Autodesk Inventor part; units mm, degrees
ref_plane "YZ Plane" through (0, 0, 0) normal (1, 0, 0) x (0, 1, 0)
ref_plane "XZ Plane" through (0, 0, 0) normal (0, 1, 0) x (-1, 0, 0)
ref_plane "XY Plane" through (0, 0, 0) normal (0, 0, 1) x (1, 0, 0)
sketch "Sketch2" plane through (0, 0, 0) normal (0, 0, 1) x (1, 0, 0)
  arc A0 (0, -52) -> (0, 52) centre (0, 0) ccw
  arc A1 (0, -50) -> (0, 50) centre (0, 0) ccw
  line L0 (0, 52) -> (0, 50)
  line L1 (0, -50) -> (0, -52)
  line L2 (2, 49.96) -> (4, 49.96)
  line L3 (4, 49.96) -> (4, 65.96)
  line L4 (4, 65.96) -> (2, 65.96)
  line L5 (2, 65.96) -> (2, 49.96)
  line L6 (2, -49.96) -> (4, -49.96)
  line L7 (4, -49.96) -> (4, -65.96)
  line L8 (4, -65.96) -> (2, -65.96)
  line L9 (2, -65.96) -> (2, -49.96)
  line L10 (0, 92.344) -> (0, -92.344) construction
  point P0 (4, -51.8459)
  point P1 (4, 51.8459)
  dimension "d0" = 104
  dimension "d1" = 100
  dimension "d2" = 2
  dimension "d40" = 2
  dimension "d41" = 2
  dimension "d42" = 16
  dimension "d43" = 16
  dimension "d44" = 2
  dimension "d45" = 2
extrude "Extrusion1" add sketch "Sketch2" along normal blind 80 contours L9 L6 L7 A0 | A0 L7 L8 L9 | L7 L6 A1 L2 L3 A0 | L3 L2 L5 A0 | A0 L5 L4 L3
fillet "Fillet4" radius 2 2 edges at (4, 51.8459, 40) (4, -51.8459, 40)
sketch "Sketch6" plane through (4, -65.96, 80) normal (1, 0, 0) x (0, 0, -1)
  line L0 (80, 16) -> (80, 0) construction
  line L1 (80, 0) -> (0, 0) construction
  line L2 (0, 16) -> (0, 0) construction
  line L3 (80, 16) -> (0, 16) construction
  line L4 (80, 131.92) -> (80, 115.92) construction
  line L5 (80, 115.92) -> (0, 115.92) construction
  line L6 (0, 131.92) -> (0, 115.92) construction
  line L7 (80, 131.92) -> (0, 131.92) construction
  point P0 (80, 65.96)
  point P1 (15, 6)
  point P2 (65, 6)
  point P3 (65, 125.92)
  point P4 (15, 125.92)
  dimension "d47" = 15
  dimension "d48" = 15
  dimension "d49" = 15
  dimension "d50" = 15
  dimension "d51" = 6
  dimension "d52" = 6
  dimension "d53" = 6
  dimension "d54" = 6
hole "Hole3" at (4, -59.96, 65) at (4, -59.96, 15) at (4, 59.96, 15) at (4, 59.96, 65) direction (-1, 0, 0) diameter 6.5 depth 2
properties part number "P050_SupportTube2"
For this review, take the finished solid that the model builds, in its own axes (mm). A direction names the side the tool comes from. Round coordinates to 2 decimals unless told otherwise and drop trailing zeros. Write each loop counter-clockwise with the first axis right and the second up, starting at its lowest first coordinate (ties: lowest second). Pieces come first, ordered by that corner, then holes. Notation, with made-up numbers: M 83,76 L 96,76 A24 cw 96,86 Z; hole C 54,70.5 d5. An arc over 180 degrees is marked long. One line per item, written item: value. Start each with the question number.
(1) We need section B-B (y = 59.96). Give the boundary of the cut face in (x, z), and give its area (3 significant figures).
(2) Insertion check: pin 1 (4 mm diameter, centred on x = 45.5, z = 17.5, fed in from +Y); pin 2 (1 mm diameter, centred on x = 46.5, z = 18.5, fed in from -Y); pin 3 (1 mm diameter, centred on y = 35.5, z = 45, fed in from +X). Each pin has a flat end and moves straight along its axis. Give the tip position at first contact, or say it passes through.
(3) We need section D-D (z = 24.5). Give the boundary of the cut face in (x, y).
(4) Wall thickness on line 1 (Z direction, x = 3.55, y = -59.96); line 2 (Y direction, x = 3.4, z = 15); line 3 (X direction, y = 53.5, z = 22.5): over which ranges is each line inside the solid? List them lowest first.
(5) Machinability: for faces 5 (the flat face through (4, -60, 39)), 6 (the cylindrical face through (2.986, -60.103, 68.247)), 7 (the flat face through (4, 60, 39)), which of the approach directions +Z, -Z, +X, -X, +Y, -Y give a long, thin tool a straight path to every point of the face, cutting with its end or side? Answer none if there is none.
(6) We need section C-C (z = 65). Give the boundary of the cut face in (x, y).
(7) We need section A-A (x = 48). Give the boundary of the cut face in (y, z), and give its area (3 significant figures).
(8) The part is to be moulded in two halves that separate along Y. For faces 1 (the cylindrical face through (49.99, 1.07, 39.44)), 2 (the flat face through (51, 0, 80)), 3 (the cylindrical face through (2.986, -62.157, 17.395)), 4 (the cylindrical face through (51.99, 1.06, 39.44)), say which applies: released by +Y, released by -Y, zero draft, split by the parting line, or undercut.
Result:
1. outline: M 2,0 L 4,0 L 4,11.75 L 2,11.75 Z; M 2,18.25 L 4,18.25 L 4,61.75 L 2,61.75 Z; M 2,68.25 L 4,68.25 L 4,80 L 2,80 Z
1. area: 134 mm²
2. pin 1: y = 28.49
2. pin 2: y = -24.25
2. pin 3: x = 38.46
3. outline: M 2,-65.96 L 4,-65.96 L 4,-53.67 A2 cw 5.78,-51.68 A52 ccw 5.78,51.68 A2 cw 4,53.67 L 4,65.96 L 2,65.96 L 2,49.96 A50 cw 2,-49.96 Z
4. line 1: 0 to 11.75, 18.25 to 61.75, 68.25 to 80
4. line 2: -65.96 to -63.21, -56.71 to -49.88, 49.88 to 56.71, 63.21 to 65.96
4. line 3: 2 to 4.01
5. face 5: +Z, -Z, +X, -Y
5. face 6: +X, -X
5. face 7: +Z, -Z, +X, +Y
6. outline: M 2,-65.96 L 4,-65.96 L 4,-63.21 L 2,-63.21 Z; M 2,-56.71 L 4,-56.71 L 4,-53.67 A2 cw 5.78,-51.68 A52 ccw 5.78,51.68 A2 cw 4,53.67 L 4,56.71 L 2,56.71 L 2,49.96 A50 cw 2,-49.96 Z; M 2,63.21 L 4,63.21 L 4,65.96 L 2,65.96 Z
7. outline: M -20,0 L -14,0 L -14,80 L -20,80 Z; M 14,0 L 20,0 L 20,80 L 14,80 Z
7. area: 960 mm²
8. face 1: undercut
8. face 2: zero draft
8. face 3: undercut
8. face 4: split by the parting line
